```python
from build123d import *

# Parameters (mm, degrees)
BOSS_EXTRUDE1_DEPTH    = 3.175
SKETCH2_R              = 17.4625
CUT_EXTRUDE1_DEPTH     = 385.384860036
F_10_CLEARANCE_HOLE1_D = 5.1054
SKETCH6_R              = 2.794
CUT_EXTRUDE2_DEPTH     = 385.384860036
SKETCH7_R              = 1.905
CUT_EXTRUDE3_DEPTH     = 385.384860036


with BuildPart() as part:
    # Sketch1 → Boss-Extrude1 (new body)
    with BuildSketch(Plane.XY):
        with BuildLine():
            Line((0, 0), (355.6, 0))
            ThreePointArc((355.6, 0), (381, 25.4), (355.6, 50.8))
            Line((355.6, 50.8), (0, 50.8))
            ThreePointArc((0, 50.8), (-25.4, 25.4), (0, 0))
        make_face()
    extrude(amount=BOSS_EXTRUDE1_DEPTH)

    # Sketch2 → Cut-Extrude1 (cut, through all)
    with BuildSketch(Plane.XY.offset(3.175)):
        with Locations((0, 25.4)):
            Circle(SKETCH2_R)
        with Locations((355.6, 25.4)):
            Circle(SKETCH2_R)
    extrude(amount=-CUT_EXTRUDE1_DEPTH, mode=Mode.SUBTRACT)

    # #10 Clearance Hole1 (through all)
    with Locations(Plane(origin=(18.257547563, 35.941, 3.175), x_dir=(1, 0, 0), z_dir=(0, 0, 1))):
        with Locations((0, 0), (0, -21.082), (-18.257547563, -31.623), (-36.515095126, -21.082), (-36.515095126, 0), (-18.257547563, 10.541)):
            Hole(F_10_CLEARANCE_HOLE1_D / 2)

    # Sketch6 → Cut-Extrude2 (cut, through all)
    with BuildSketch(Plane.XY.offset(3.175)):
        with Locations((63.5, 25.4)):
            Circle(SKETCH6_R)
        with Locations((88.9, 25.4)):
            Circle(SKETCH6_R)
        with Locations((152.4, 25.4)):
            Circle(SKETCH6_R)
        with Locations((177.8, 25.4)):
            Circle(SKETCH6_R)
    extrude(amount=-CUT_EXTRUDE2_DEPTH, mode=Mode.SUBTRACT)

    # Sketch7 → Cut-Extrude3 (cut, through all)
    with BuildSketch(Plane.XY.offset(3.175)):
        with Locations((258.687715098, 40.64)):
            Circle(SKETCH7_R)
        with Locations((245.987715098, 40.64)):
            Circle(SKETCH7_R)
        with Locations((233.287715098, 40.64)):
            Circle(SKETCH7_R)
    extrude(amount=-CUT_EXTRUDE3_DEPTH, mode=Mode.SUBTRACT)


solid = part.part
```
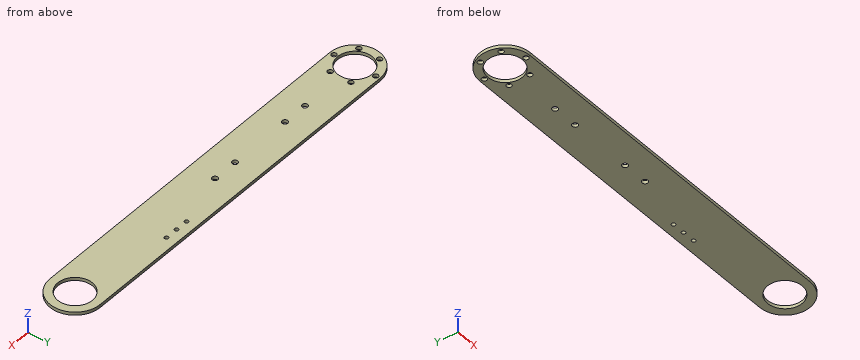
The model under review builds one solid part; all positions refer to its coordinate system, in mm. Round coordinates to 2 decimals unless told otherwise and drop trailing zeros. Loops run counter-clockwise (first coordinate to the right, second up) from the corner with the lowest first, then second, coordinate; pieces in that order, holes last. Notation, with made-up numbers: (23, -31) -> (64, -31) arc R31 ccw to (64, -1) -> close; hole circle Ø3 at (-11, -32.5). An arc over 180 degrees is marked (long way). Answer as a JSON object with one key per item and string values. Group by question number.
1) For pin 1 Ø8 at (x, y) = (-18.26, 14.86) entering from +Z (3 decimals), flat-tipped, find the tip position at first contact; note if it passes through.
2) We need section A-A on x = 345.5. Write out the cut boundary in (y, z) (3 decimals), then the cut area to 3 significant figures.
3) For line 1 (X direction, y = 39.5, z = 1.15); line 2 (X direction, y = 38, z = 0.45); line 3 (X direction, y = 15, z = 1.6), list the stretches that pass through material, from the lowest coordinate up. Write a range as [from, to].
4) We need section B-B on z = 1.75. Give the number of separate pieces and of enclosed holes in the cut face, then the cut area to 3 significant figures.
Result set:
{
 "1": {"pin 1": "z = 3.175"},
 "2": {"outline": "(0, 0) -> (11.155, 0) -> (11.155, 3.175) -> (0, 3.175) -> close; (39.645, 0) -> (50.8, 0) -> (50.8, 3.175) -> (39.645, 3.175) -> close", "area": "70.8 mm²"},
 "3": {"line 1": "[-21.13, -10.3], [10.3, 231.76], [234.81, 244.46], [247.51, 257.16], [260.21, 345.3], [365.9, 376.73]", "line 2": "[-22.05, -19.77], [-16.75, -12.09], [12.09, 16.75], [19.77, 343.51], [367.69, 377.65]", "line 3": "[-23.17, -20.81], [-15.71, -14.03], [14.03, 15.71], [20.81, 341.57], [369.63, 378.77]"},
 "4": {"separate pieces": "1", "enclosed holes": "15", "area": "17,900 mm²"}
}
